Read the model definition and answer for the solid it produces. Units are mm, in the model's axes. A direction names the side the tool comes from. Coordinates: 2 decimals unless noted, no trailing zeros. Order: outer loops, then holes, each group sorted by start corner. A loop starts at its lowest first (then second) coordinate and runs counter-clockwise, first axis right, second up. Notation, with made-up numbers: (34.25, 69) - (76.25, 69) arc R12 cw to (76.25, 85) - close; hole circle Ø2 at (-32.75, -10.5). An arc over 180 degrees is marked (long way). Write item = value, one per line.
from build123d import *

# Parameters (mm, degrees)
F1_DEPTH = 393.7
F2_R     = 5.08
F4_DEPTH = 76.2
F6_DEPTH = 25.4


with BuildPart() as f1:
    # F0 (on Front) → F1 (new body, symmetric)
    with BuildSketch(Plane.XZ):
        Polygon((-38.1, -38.1), (38.1, -38.1), (38.1, -31.75), (-31.75, -31.75), (-31.75, 38.1), (-38.1, 38.1), align=None)
    extrude(amount=F1_DEPTH, both=True)

    # F2
    f2_edges = [f1.edges().sort_by_distance(p)[0] for p in [
        (-31.75, 0, 38.1),
        (-31.75, 0, -31.75),
        (38.1, 0, -31.75),
    ]]
    fillet(f2_edges, radius=F2_R)

    # F3 (on face) → F4 (cut)
    with BuildSketch(Plane(origin=(0, 0, -38.1), x_dir=(1, 0, 0), z_dir=(0, 0, -1))):
        Polygon((-38.1, -393.7), (38.1, -393.7), (-38.1, -317.5), align=None)
    extrude(amount=-F4_DEPTH, mode=Mode.SUBTRACT)

    # F5 (on face) → F6 (cut)
    with BuildSketch(Plane.YZ.offset(-31.75)):
        Polygon((200.3282578849, 46.1080149466), (323.85, -40.3828400151), (323.85, 46.1080149466), align=None)
    extrude(amount=-F6_DEPTH, mode=Mode.SUBTRACT)


solid = f1.part
1) For faces 1 (the face through (-1, -6, -38.1)), 2 (the face through (4, -8, -31.75)), determine the directions among +Z, -Z, +X, -X, +Y, -Y from which every point of the face is accessible in a straight line to the end or side of a thin tool.
Returned:
face_1 = -Z, +X, -X, +Y, -Y
face_2 = +Z, +X, +Y, -Y
2) Flat-ended cylindrical pins translate along their axes: pin 1 Ø4 at (y, z) = (-15, -11.5) entering from +X; pin 2 Ø8 at (x, z) = (29.5, -30.5) entering from +Y; pin 3 Ø5.5 at (y, z) = (318, -34.5) entering from -X. Find the tip coordinate at first contact, or state that the pin passes through.
Returned:
pin_1 = -31.75
pin_2 = 388.9
pin_3 = -38.1
3) Straight lines are drawn through the part: line 1 along X through (y, z) = (165, 31); line 2 along Y through (x, z) = (-32, -18). For each, find the intervals that lie inside material, in ascending order. Write a range as from..to.
Returned:
line_1 = -38.1..-31.75
line_2 = -393.7..291.88
4) The part is cut by section B-B (x = 19). Determine the outline of the cut face in (y, z), and give its area (3 significant figures).
Returned:
outline = (-393.7, -38.1) - (374.6, -38.1) - (374.6, -31.75) - (-393.7, -31.75) - close
area = 4,880 mm^2
5) The part is cut by section C-C (z = 19.5). Determine the outline of the cut face in (x, y).
Returned:
outline = (-38.1, -393.7) - (-31.75, -393.7) - (-31.75, 238.33) - (-38.1, 238.33) - close
6) The part is cut by section A-A (y = -57.5). Determine the outline of the cut face in (x, z), and give its area (3 significant figures).
Returned:
outline = (-38.1, -38.1) - (38.1, -38.1) - (38.1, -36.83) arc R5.08 ccw to (33.02, -31.75) - (-26.67, -31.75) arc R5.08 cw to (-31.75, -26.67) - (-31.75, 33.02) arc R5.08 ccw to (-36.83, 38.1) - (-38.1, 38.1) - close
area = 922 mm^2
